Here's how the part is built. I have some questions about the finished solid (model axes, mm). A direction names the side the tool comes from. Give positions to 0.01 mm unless a question says otherwise; leave off trailing zeros. Order: outer loops, then holes, each group sorted by start corner. A loop starts at its lowest first (then second) coordinate and runs counter-clockwise, first axis right, second up. Notation, with made-up numbers: (55.25, 88) -> (102.25, 88) arc R36 ccw to (102.25, 122) -> close; hole circle Ø7 at (15, 42). An arc over 180 degrees is marked (long way). Write each question's results on one line, items separated by ' | '. Start each with the question number.
Q1. Imagine slicing it at D-D, the plane x = 15. Please give me the cut outline in (y, z).
Q2. I need wall thicknesses on line 1 along X through (y, z) = (1.5, 1.1); line 2 along X through (y, z) = (-5, 0.9); line 3 along Y through (x, z) = (-23, 3.9). Which ranges of each line are inside material? Lowest first, please. Write a range as [from, to].
Q3. I'm going to push flat-ended pins straight in: pin 1 (10.5 mm diameter, centred on x = 0, y = 0, fed in from +Z); pin 2 (1 mm diameter, centred on x = 5.5, z = 2.5, fed in from -Y); pin 3 (1 mm diameter, centred on x = 16.5, z = 5, fed in from -Y). Where does each tip first touch, or does it pass through?
Q4. Imagine slicing it at A-A, the plane x = 23. Please give me the cut outline in (y, z).
Q5. Imagine slicing it at B-B, the plane z = 3.15. Please give me the cut outline in (x, y), then the cut area to 3 significant figures.
Q6. For faces 5 (the face through (20, 8, 3)), 6 (the face through (-7.1, -5.45, 5.06)), 7 (the face through (-20, -8, 3)), which set-ups out of +Z, -Z, +X, -X, +Y, -Y let a thin tool reach every point of the face, with its end or its side?
Q7. Thinking about a two-plate mould opening in X: for faces 1 (the face through (7, -8, 6)), 2 (the face through (0, 0, 2)), 3 (the face through (-30.556, 0, 3)), 4 (the face through (-20.77, 0.74, 2.96)), which applies, pulls with the +X half, pulls with the -X half, needs draft (parallel to the pull), parting line crosses it, or undercut?
```python
from build123d import *

# Parameters (mm, degrees)
F0_R     = 2.45
F1_DEPTH = 6
F2_R     = 8.95
F3_DEPTH = 4
F4_R     = 2.1
F5_R     = 0.4
F6_DEPTH = 2.001


with BuildPart() as f1:
    # F0 (on Top) → F1 (new body)
    with BuildSketch(Plane.XY):
        with BuildLine():
            ThreePointArc((8.944272, -8), (11.210068, -4.281865), (12, 0))
            ThreePointArc((12, 0), (11.210068, 4.281865), (8.944272, 8))
            ThreePointArc((8.944272, 8), (0, 12), (-8.944272, 8))
            ThreePointArc((-8.944272, 8), (-12, 0), (-8.944272, -8))
            ThreePointArc((-8.944272, -8), (0, -12), (8.944272, -8))
        make_face()
        with BuildLine():
            ThreePointArc((8.944272, 8), (11.210068, 4.281865), (12, 0))
            ThreePointArc((12, 0), (11.210068, -4.281865), (8.944272, -8))
            Line((8.944272, -8), (31.067557, -8))
            Line((31.067557, -8), (31.067557, 8))
            Line((31.067557, 8), (8.944272, 8))
        make_face()
        with Locations((23.617557, 0)):
            Circle(F0_R, mode=Mode.SUBTRACT)
        with BuildLine():
            ThreePointArc((-8.944272, -8), (-12, 0), (-8.944272, 8))
            Line((-8.944272, 8), (-30.555639, 8))
            Line((-30.555639, 8), (-30.555639, -8))
            Line((-30.555639, -8), (-8.944272, -8))
        make_face()
        with Locations((-23.105639, 0)):
            Circle(F0_R, mode=Mode.SUBTRACT)
    extrude(amount=F1_DEPTH)

    # F2 (on face) → F3 (cut)
    with BuildSketch(Plane.XY.offset(6)):
        Circle(F2_R)
    extrude(amount=-F3_DEPTH, mode=Mode.SUBTRACT)

    # F4
    f4_edges = [f1.edges().sort_by_distance(p)[0] for p in [
        (-8.95, 0, 2),
    ]]
    fillet(f4_edges, radius=F4_R)

    # F5 (on face) → F6 (cut, through all)
    with BuildSketch(Plane.XY.offset(2)):
        with Locations((-5.35, 0)):
            Circle(F5_R)
        with Locations((-4.500706, -2.892428)):
            Circle(F5_R)
        with Locations((-2.22247, -4.866531)):
            Circle(F5_R)
        with Locations((0.761384, -5.295545)):
            Circle(F5_R)
        with Locations((3.503505, -4.04326)):
            Circle(F5_R)
        with Locations((5.133287, -1.507269)):
            Circle(F5_R)
        with Locations((5.133287, 1.507269)):
            Circle(F5_R)
        with Locations((3.503505, 4.04326)):
            Circle(F5_R)
        with Locations((0.761384, 5.295545)):
            Circle(F5_R)
        with Locations((-2.22247, 4.866531)):
            Circle(F5_R)
        with Locations((-4.500706, 2.892428)):
            Circle(F5_R)
    extrude(amount=-F6_DEPTH, mode=Mode.SUBTRACT)


solid = f1.part
```
Geometry check:
1) outline: (-8, 0) -> (8, 0) -> (8, 6) -> (-8, 6) -> close
2) line 1: [-30.56, -25.04], [-21.17, 4.73], [5.53, 21.68], [25.55, 31.07] | line 2: [-30.56, -2.6], [-1.85, 0.49], [1.03, 31.07] | line 3: [-8, -2.45], [2.45, 8]
3) pin 1: z = 2 | pin 2: y = -10.91 | pin 3: y = -8
4) outline: (-8, 0) -> (-2.37, 0) -> (-2.37, 6) -> (-8, 6) -> close; (2.37, 0) -> (8, 0) -> (8, 6) -> (2.37, 6) -> close
5) outline: (-30.56, -8) -> (-8.94, -8) arc R12 ccw to (8.94, -8) -> (31.07, -8) -> (31.07, 8) -> (8.94, 8) arc R12 ccw to (-8.94, 8) -> (-30.56, 8) -> close; hole circle Ø4.9 at (-23.11, 0); hole circle Ø17.45 at (0, 0); hole circle Ø4.9 at (23.62, 0) | area: 808 mm²
6) face 5: +Z, -Z, +X, +Y | face 6: +Z | face 7: +Z, -Z, -X, -Y
7) face 1: needs draft | face 2: undercut | face 3: pulls with the -X half | face 4: undercut
